Could you check a few things on this model? Use its own coordinates, in mm. A direction names the side the tool comes from. Round coordinates to 2 decimals unless told otherwise and drop trailing zeros. Loops run counter-clockwise (first coordinate to the right, second up) from the corner with the lowest first, then second, coordinate; pieces in that order, holes last.
from build123d import *

# Parameters (mm, degrees)
SKETCH1_W           = 28
SKETCH1_H           = 16
BOSS_EXTRUDE1_DEPTH = 19.2
SKETCH2_W           = 0.75
SKETCH2_H           = 6.4
BOSS_EXTRUDE2_DEPTH = 10.2
SKETCH3_W           = 6.3
SKETCH3_H           = 0.85
BOSS_EXTRUDE3_DEPTH = 8.45
BOSS_EXTRUDE4_DEPTH = 14
SKETCH5_R           = 3.5
BOSS_EXTRUDE5_DEPTH = 18.5


with BuildPart() as part:
    # Sketch1 → Boss-Extrude1 (new body)
    with BuildSketch(Plane(origin=(0, 0, 0), x_dir=(1, 0, 0), z_dir=(0, 1, 0))):
        with Locations((-14, 8)):
            Rectangle(SKETCH1_W, SKETCH1_H)
    extrude(amount=BOSS_EXTRUDE1_DEPTH)

    # Sketch2 → Boss-Extrude2 (add)
    with BuildSketch(Plane.XZ):
        with Locations((-1.625, -8)):
            Rectangle(SKETCH2_W, SKETCH2_H)
        with Locations((-26.375, -8)):
            Rectangle(SKETCH2_W, SKETCH2_H)
    extrude(amount=BOSS_EXTRUDE2_DEPTH)

    # Sketch3 → Boss-Extrude3 (add)
    with BuildSketch(Plane.ZY.offset(28)):
        with Locations((-4.85, 16.145)):
            Rectangle(SKETCH3_W, SKETCH3_H)
    extrude(amount=BOSS_EXTRUDE3_DEPTH)

    # Sketch4 → Boss-Extrude4 (add)
    with BuildSketch(Plane(origin=(0, 19.2, 0), x_dir=(1, 0, 0), z_dir=(0, 1, 0))):
        with BuildLine():
            ThreePointArc((-8.790541147, 10.97683363), (-16.97683363, 13.209458853), (-19.209458853, 5.02316637))
            Line((-19.209458853, 5.02316637), (-8.790541147, 10.97683363))
        make_face()
        with BuildLine():
            Line((-8.790541147, 10.97683363), (-19.209458853, 5.02316637))
            ThreePointArc((-19.209458853, 5.02316637), (-12.459992389, 2.201002107), (-8, 8))
            ThreePointArc((-8, 8), (-8.201002107, 9.540007611), (-8.790541147, 10.97683363))
        make_face()
    extrude(amount=BOSS_EXTRUDE4_DEPTH)

    # Sketch5 → Boss-Extrude5 (add)
    with BuildSketch(Plane(origin=(0, 33.2, 0), x_dir=(1, 0, 0), z_dir=(0, 1, 0))):
        with Locations(Location((-14, 8, 0), (0, 0, 270))):
            Circle(SKETCH5_R)
    extrude(amount=BOSS_EXTRUDE5_DEPTH)


solid = part.part
Item 1: If we section it at A-A, the plane x = -14: Please give me the cut outline in (y, z).
Results list:
outline: (0, -16) - (19.2, -16) - (19.2, -14) - (33.2, -14) - (33.2, -11.5) - (51.7, -11.5) - (51.7, -4.5) - (33.2, -4.5) - (33.2, -2) - (19.2, -2) - (19.2, 0) - (0, 0) - close
Item 2: If we section it at B-B, the plane y = 24.5: Please give me the cut outline in (x, z), then the cut area to 3 significant figures.
Results list:
outline: circle Ø12 at (-14, -8)
area: 113 mm2
Item 3: We'd pull the mould along X, two halves only. Please class faces 1 (the flat face through (-14, 0, -8)), 2 (the flat face through (-26.75, -5, -8)), 3 (the flat face through (-17.3, 19.2, -13.4)): released by +X, released by -X, zero draft, split by the parting line, or undercut.
Results list:
face 1: undercut
face 2: released by -X
face 3: zero draft
Item 4: For faces 4 (the flat face through (-32, 16.57, -5)), 5 (the flat face through (-2, -5, -8)), 6 (the flat face through (-1.25, -5, -8)), 7 (the flat face through (-32, 15.72, -5)), 8 (the flat face through (-11, 33.2, -5)), which set-ups out of +Z, -Z, +X, -X, +Y, -Y let a thin tool reach every point of the face, with its end or its side?
Results list:
face 4: +Z, -Z, -X, +Y
face 5: +Z, -Z, -Y
face 6: +Z, -Z, +X, -Y
face 7: +Z, -Z, -X, -Y
face 8: +Y
Item 5: If we section it at C-C, the plane z = -7.25: Please give me the cut outline in (x, y), then the cut area to 3 significant figures.
Results list:
outline: (-36.45, 15.72) - (-28, 15.72) - (-28, 0) - (-26.75, 0) - (-26.75, -10.2) - (-26, -10.2) - (-26, 0) - (-2, 0) - (-2, -10.2) - (-1.25, -10.2) - (-1.25, 0) - (0, 0) - (0, 19.2) - (-8.05, 19.2) - (-8.05, 33.2) - (-10.58, 33.2) - (-10.58, 51.7) - (-17.42, 51.7) - (-17.42, 33.2) - (-19.95, 33.2) - (-19.95, 19.2) - (-28, 19.2) - (-28, 16.57) - (-36.45, 16.57) - close
area: 853 mm2
Item 6: If we section it at D-D, the plane x = -31: Please give me the cut outline in (y, z).
Results list:
outline: (15.72, -8) - (16.57, -8) - (16.57, -1.7) - (15.72, -1.7) - close
Item 7: Will these pins go through, and if not, where does the flat tip stop? pin 1 (1.9 mm diameter, centred on x = -30.5, z = -6, fed in from +Y); pin 2 (2 mm diameter, centred on x = -23, z = -2, fed in from -Y); pin 3 (3 mm diameter, centred on y = -4, z = -8.5, fed in from -X); pin 4 (1 mm diameter, centred on y = 6.5, z = -13, fed in from +X).
Results list:
pin 1: stops at y = 16.57
pin 2: stops at y = 0
pin 3: stops at x = -26.75
pin 4: stops at x = 0
Item 8: If I drill on line 1 along X through (y, z) = (-0.5, -7.25); line 2 along Y through (x, z) = (-7.5, -15); line 3 along Y through (x, z) = (-17, -6.25), over which ranges is the centre line in solid material (lowest first)?
Results list:
line 1: x = -26.75 to -26, -2 to -1.25
line 2: y = 0 to 19.2
line 3: y = 0 to 51.7
